Geometry check sheet. Reference: drawing and pictorial views, mm from the part's lowest x, y, z. A direction names the side the tool comes from. Round coordinates to 2 decimals unless told otherwise and drop trailing zeros. Write each loop counter-clockwise with the first axis right and the second up, starting at its lowest first coordinate (ties: lowest second). Pieces come first, ordered by that corner, then holes. Notation, with made-up numbers: M 76,-25 L 89,-25 A26 cw 89,7 Z; hole C 38,43 d10. An arc over 180 degrees is marked long. Answer in a Markdown table with one row per item.
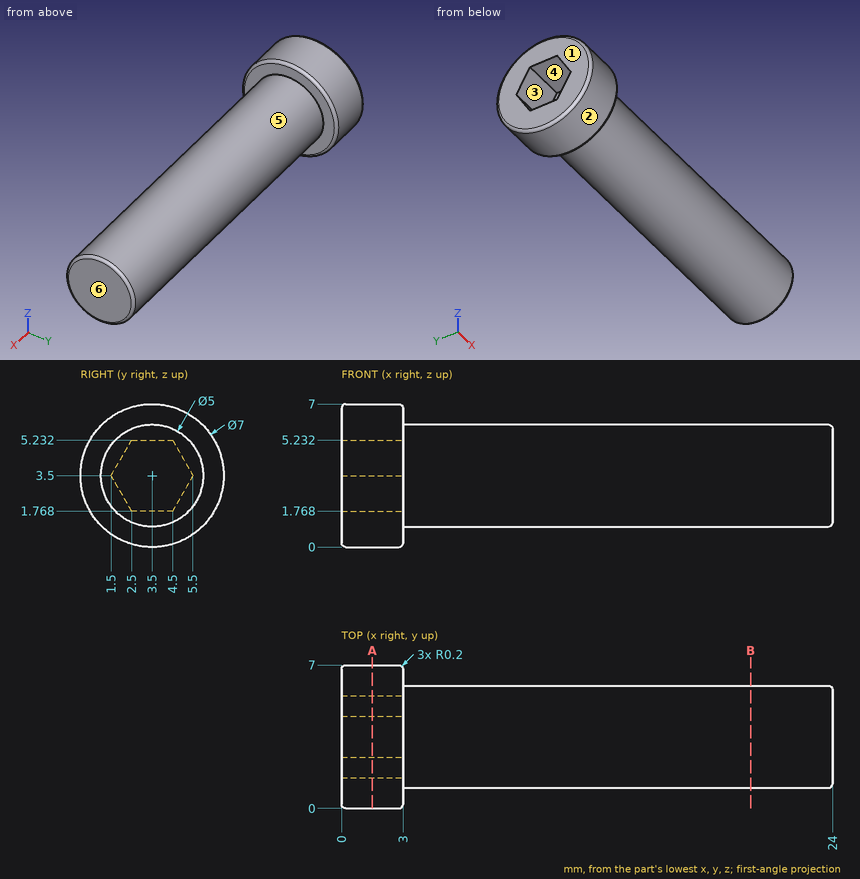
1. Scan lines: L1, parallel to X at y = 5.75, z = 1.5; L2, parallel to Z at x = 21.5, y = 5. Record each from-to range of solid material in increasing order.
Found:
| item | result |
|---|---|
| L1 | x = 0 to 3 |
| L2 | z = 1.5 to 5.5 |
2. Section check A-A, the plane x = 1.5. Record the cut outline in (y, z), and give its area (3 significant figures).
Found:
| item | result |
|---|---|
| outline | C 3.5,3.5 d7; hole M 1.5,3.5 L 2.5,1.77 L 4.5,1.77 L 5.5,3.5 L 4.5,5.23 L 2.5,5.23 Z |
| area | 28.1 mm2 |
3. Go/stop test with flat-tipped pins: pin 1 (2 mm diameter, centred on x = 12, z = 3, fed in from -Y); pin 2 (4 mm diameter, centred on y = 5.5, z = 6, fed in from -X); pin 3 (1.5 mm diameter, centred on x = 7, z = 6, fed in from -Y); pin 4 (1 mm diameter, centred on y = 4, z = 3, fed in from -X). Record where each tip stops, or that it passes through.
Found:
| item | result |
|---|---|
| pin 1 | stops at y = 1 |
| pin 2 | stops at x = 0 |
| pin 3 | stops at y = 1.71 |
| pin 4 | stops at x = 3 |
4. Draft check along Y on the marked faces 1, 2 and 3. Enter one of: +Y half, -Y half, draft (parallel to the pull), parting line (faces both ways), or undercut.
Found:
| item | result |
|---|---|
| face 1 | draft |
| face 2 | parting line |
| face 3 | undercut |
5. Access from +Z, -Z, +X, -X, +Y, -Y to the whole of each face (thin tool, end or side, straight path). Record for the marked faces 4, 5 and 6.
Found:
| item | result |
|---|---|
| face 4 | -X |
| face 5 | +X |
| face 6 | +Z, -Z, +X, +Y, -Y |
6. Section check B-B, the plane x = 20. Record the cut outline in (y, z).
Found:
| item | result |
|---|---|
| outline | C 3.5,3.5 d5 |
